Here's how the part is built. I have some questions about the finished solid (model axes, mm). Face numbers are marked on the shaded views. A direction names the side the tool comes from. Coordinates: 2 decimals unless noted, no trailing zeros. Write each loop counter-clockwise with the first axis right and the second up, starting at its lowest first coordinate (ties: lowest second). Pieces come first, ordered by that corner, then holes.
Item 1: If we section it at C-C (x = 50.5): Please give me the cut outline in (y, z), then the cut area to 3 significant figures.
Item 2: If we section it at D-D (z = -9): Please give me the cut outline in (x, y), then the cut area to 3 significant figures.
Item 3: If we section it at B-B (z = -17.5): Please give me the cut outline in (x, y).
Item 4: For the marked faces 1, 2 and 3, which set-ups out of +Z, -Z, +X, -X, +Y, -Y let a thin tool reach every point of the face, with its end or its side?
Item 5: I'm going to push flat-ended pins straight in: pin 1 Ø0.8 at (x, z) = (57.5, -31.5) entering from -Y; pin 2 Ø1.4 at (x, z) = (34.5, -18) entering from +Y; pin 3 Ø3 at (x, y) = (37, -489.5) entering from -Z. Where does each tip first touch, or does it pass through?
Item 6: We'd pull the mould along Y, two halves only. Please class the marked faces 4, 5, 6 and 7: +Y half, -Y half, draft (parallel to the pull), parting line (faces both ways), or undercut.
Item 7: If I drill on line 1 (X direction, y = -492, z = -33.1); line 2 (Z direction, x = 60, y = -548); line 3 (X direction, y = -536.7, z = -8), over which ranges is the centre line in solid material (lowest first)?
Item 8: If we section it at A-A (y = -536.7): Please give me the cut outline in (x, z).
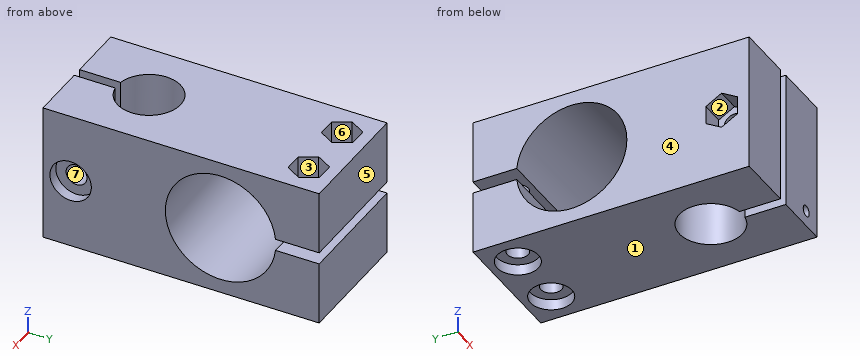
from build123d import *

# Parameters (mm, degrees)
BOSS_EXTRU_1_DEPTH                               = 35
BOSS_EXTRU_2_DEPTH                               = 31.5
CHAMBRAGE_POUR_VIS_T_TE_RONDE_6_PANS_D           = 5.3
CHAMBRAGE_POUR_VIS_T_TE_RONDE_6_PANS_DEPTH       = 44
CHAMBRAGE_POUR_VIS_T_TE_RONDE_6_PANS_CBORE_D     = 10.5
CHAMBRAGE_POUR_VIS_T_TE_RONDE_6_PANS_CBORE_DEPTH = 2.75
CHAMBRAGE_POUR_VIS_T_TE_RONDE_6_PANS_TIP         = 1.59228064
ENL_V_MAT_EXTRU_1_DEPTH                          = 8
ENL_V_MAT_EXTRU_2_DEPTH                          = 45
CHAMBRAGE_POUR_VIS_T_TE_RONDE_6_2_D              = 5.3
CHAMBRAGE_POUR_VIS_T_TE_RONDE_6_2_DEPTH          = 44
CHAMBRAGE_POUR_VIS_T_TE_RONDE_6_2_CBORE_D        = 10.5
CHAMBRAGE_POUR_VIS_T_TE_RONDE_6_2_CBORE_DEPTH    = 2.75
CHAMBRAGE_POUR_VIS_T_TE_RONDE_6_2_TIP            = 1.59228064
ENL_V_MAT_EXTRU_3_DEPTH                          = 6
ESQUISSE12_R                                     = 1.4
ENL_V_MAT_EXTRU_4_DEPTH                          = 5


with BuildPart() as part:
    # Esquisse1 → Boss.-Extru.1 (new body)
    with BuildSketch(Plane.XY):
        with BuildLine():
            Line((47.415392001, -544.601740315), (47.415392001, -555))
            Line((47.415392001, -555), (61.915392001, -555))
            Line((61.915392001, -555), (61.915392001, -505))
            Line((61.915392001, -505), (30.415392001, -505))
            Line((30.415392001, -505), (30.415392001, -555))
            Line((30.415392001, -555), (44.915392001, -555))
            Line((44.915392001, -555), (44.915392001, -544.601740315))
            ThreePointArc((44.915392001, -544.601740315), (46.165392001, -528.7), (47.415392001, -544.601740315))
        make_face()
    extrude(amount=-BOSS_EXTRU_1_DEPTH)

    # Esquisse4 → Boss.-Extru.2 (add)
    with BuildSketch(Plane(origin=(61.915392001, 0, 0), x_dir=(0, 0, -1), z_dir=(1, 0, 0))):
        Polygon((35, -505), (35, -485), (19.003014107, -485), (16.003014107, -485), (0, -485), (0, -505), align=None)
    extrude(amount=-BOSS_EXTRU_2_DEPTH)

    # Chambrage pour Vis _ t_te ronde _ 6 pans
    with Locations(Plane(origin=(0, 0, -35), x_dir=(-1, 0, 0), z_dir=(0, 0, -1))):
        with Locations((-53.915392001, -492), (-38.415392001, -492)):
            CounterBoreHole(CHAMBRAGE_POUR_VIS_T_TE_RONDE_6_PANS_D / 2, CHAMBRAGE_POUR_VIS_T_TE_RONDE_6_PANS_CBORE_D / 2, CHAMBRAGE_POUR_VIS_T_TE_RONDE_6_PANS_CBORE_DEPTH, depth=CHAMBRAGE_POUR_VIS_T_TE_RONDE_6_PANS_DEPTH)
            with Locations((0, 0, -(CHAMBRAGE_POUR_VIS_T_TE_RONDE_6_PANS_DEPTH + CHAMBRAGE_POUR_VIS_T_TE_RONDE_6_PANS_TIP / 2))):  # 118° drill point
                Cone(0, CHAMBRAGE_POUR_VIS_T_TE_RONDE_6_PANS_D / 2, CHAMBRAGE_POUR_VIS_T_TE_RONDE_6_PANS_TIP, mode=Mode.SUBTRACT)

    # Esquisse7 → Enlèv. mat.-Extru.1 (cut)
    with BuildSketch(Plane.XY):
        Polygon((56.224793078, -488), (51.605990924, -488), (49.296589847, -492), (51.605990924, -496), (56.224793078, -496), (58.534194154, -492), align=None)
        Polygon((40.724793078, -488), (36.105990924, -488), (33.796589847, -492), (36.105990924, -496), (40.724793078, -496), (43.034194154, -492), align=None)
    extrude(amount=-ENL_V_MAT_EXTRU_1_DEPTH, mode=Mode.SUBTRACT)

    # Esquisse8 → Enlèv. mat.-Extru.2 (cut)
    with BuildSketch(Plane(origin=(61.915392001, 0, 0), x_dir=(0, 0, -1), z_dir=(1, 0, 0))):
        with BuildLine():
            Line((16.003014107, -485), (16.003014107, -496.080264613))
            ThreePointArc((16.003014107, -496.080264613), (17.496968442, -523.999999672), (19.003014107, -496.080914233))
            Line((19.003014107, -496.080914233), (19.003014107, -485))
            Line((19.003014107, -485), (16.003014107, -485))
        make_face()
    extrude(amount=-ENL_V_MAT_EXTRU_2_DEPTH, mode=Mode.SUBTRACT)

    # Chambrage pour Vis _ t_te ronde _ 6  2
    with Locations(Plane(origin=(61.915392001, 0, 0), x_dir=(0, 0, -1), z_dir=(1, 0, 0))):
        with Locations((17.5, -548)):
            CounterBoreHole(CHAMBRAGE_POUR_VIS_T_TE_RONDE_6_2_D / 2, CHAMBRAGE_POUR_VIS_T_TE_RONDE_6_2_CBORE_D / 2, CHAMBRAGE_POUR_VIS_T_TE_RONDE_6_2_CBORE_DEPTH, depth=CHAMBRAGE_POUR_VIS_T_TE_RONDE_6_2_DEPTH)
            with Locations((0, 0, -(CHAMBRAGE_POUR_VIS_T_TE_RONDE_6_2_DEPTH + CHAMBRAGE_POUR_VIS_T_TE_RONDE_6_2_TIP / 2))):  # 118° drill point
                Cone(0, CHAMBRAGE_POUR_VIS_T_TE_RONDE_6_2_D / 2, CHAMBRAGE_POUR_VIS_T_TE_RONDE_6_2_TIP, mode=Mode.SUBTRACT)

    # Esquisse11 → Enlèv. mat.-Extru.3 (cut)
    with BuildSketch(Plane.ZY.offset(-30.415392001)):
        Polygon((-15.190598923, -544), (-19.809401077, -544), (-22.118802154, -548), (-19.809401077, -552), (-15.190598923, -552), (-12.881197846, -548), align=None)
    extrude(amount=-ENL_V_MAT_EXTRU_3_DEPTH, mode=Mode.SUBTRACT)

    # Esquisse12 → Enlèv. mat.-Extru.4 (cut)
    with BuildSketch(Plane.XZ.offset(555)):
        with Locations(Location((56.915392001, -31, 0), (0, 0, 270))):
            Circle(ESQUISSE12_R)
    extrude(amount=-ENL_V_MAT_EXTRU_4_DEPTH, mode=Mode.SUBTRACT)


solid = part.part
Answer list:
1. outline: (-555, -35) - (-543.42, -35) - (-543.42, 0) - (-555, 0) - close; (-529.98, -35) - (-495.99, -35) - (-495.99, -32.25) - (-488.01, -32.25) - (-488.01, -35) - (-485, -35) - (-485, -19) - (-496.08, -19) arc R14 cw (long way) to (-496.08, -16) - (-485, -16) - (-485, 0) - (-489.92, 0) - (-489.92, -8) - (-494.08, -8) - (-494.08, 0) - (-529.98, 0) - close; hole circle Ø5.3 at (-548, -17.5)
1. area: 1,250 mm2
2. outline: (30.42, -555) - (44.92, -555) - (44.92, -544.6) arc R8 cw (long way) to (47.42, -544.6) - (47.42, -555) - (61.92, -555) - (61.92, -521.12) - (30.42, -521.12) - close; (30.42, -498.88) - (61.92, -498.88) - (61.92, -485) - (30.42, -485) - close; hole circle Ø5.3 at (38.42, -492); hole circle Ø5.3 at (53.92, -492)
2. area: 1,230 mm2
3. outline: (30.42, -555) - (44.92, -555) - (44.92, -550.65) - (36.42, -550.65) - (36.42, -552) - (30.42, -552) - close; (30.42, -544) - (36.42, -544) - (36.42, -545.35) - (44.92, -545.35) - (44.92, -544.6) arc R8 cw (long way) to (47.42, -544.6) - (47.42, -545.35) - (59.17, -545.35) - (59.17, -542.75) - (61.92, -542.75) - (61.92, -524) - (30.42, -524) - close; (47.42, -555) - (61.92, -555) - (61.92, -553.25) - (59.17, -553.25) - (59.17, -550.65) - (47.42, -550.65) - close
4. face 1: -Z, +X, -X, +Y, -Y
4. face 2: -X
4. face 3: +Z
5. pin 1: stops at y = -550
5. pin 2: stops at y = -523.95
5. pin 3: stops at z = -32.25
6. face 4: draft
6. face 5: +Y half
6. face 6: undercut
6. face 7: undercut
7. line 1: x = 30.42 to 33.17, 43.67 to 48.67, 59.17 to 61.92
7. line 2: z = -35 to -22.75, -12.25 to 0
7. line 3: x = 30.42 to 38.17, 54.17 to 61.92
8. outline: (30.42, -35) - (38.17, -35) - (38.17, 0) - (30.42, 0) - close; (54.17, -35) - (61.92, -35) - (61.92, 0) - (54.17, 0) - close
